The figure shows three views and two pictorial views of one solid part (mm, origin at its lowest corner). Answer the questions. Give positions to 0.01 mm unless a question says otherwise; leave off trailing zeros. Order: outer loops, then holes, each group sorted by start corner. A loop starts at its lowest first (then second) coordinate and runs counter-clockwise, first axis right, second up. Notation, with made-up numbers: M 32,13 L 61,13 A34 ccw 61,43 Z; hole C 70,86.25 d1. An arc over 180 degrees is marked long. Write item = value, one per line. Start each with the question number.
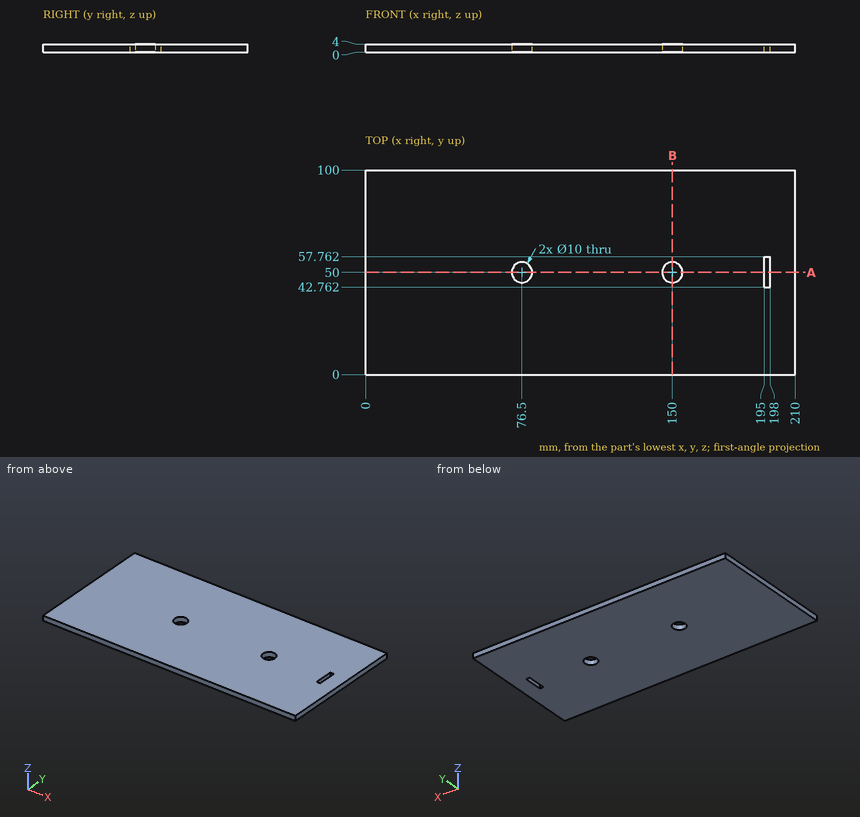
1) Find section A-A on y = 50. Determine the outline of the cut face in (x, z).
2) Find section B-B on x = 150. Determine the outline of the cut face in (y, z), plus the area to 3 significant figures.
3) This flat-tipped pin is pushed along its axis until it touches: P1, Ø8, axis at x = 150, y = 50, coming from the -Z side. Where does it stop, or does it pass through?
4) Find the intervals of material crossed by probe 1 along X at (y, z) = (55.5, 1.05); probe 2 along X at (y, z) = (53.5, 0.7); probe 3 along Y at (x, z) = (150, 1.65), in increasing order. Write a range as [from, to].
Numbers:
q1.outline = M 0,0 L 71.5,0 L 71.5,4 L 0,4 Z; M 81.5,0 L 145,0 L 145,4 L 81.5,4 Z; M 155,0 L 195,0 L 195,4 L 155,4 Z; M 198,0 L 210,0 L 210,4 L 198,4 Z
q2.outline = M 0,0 L 45,0 L 45,4 L 0,4 Z; M 55,0 L 100,0 L 100,4 L 55,4 Z
q2.area = 360 mm2
q3.P1 = through
q4.probe_1 = [0, 195], [198, 210]
q4.probe_2 = [0, 72.93], [80.07, 146.43], [153.57, 195], [198, 210]
q4.probe_3 = [0, 45], [55, 100]
